Read the model definition and answer for the solid it produces. Units are mm, in the model's axes. A direction names the side the tool comes from. Round coordinates to 2 decimals unless told otherwise and drop trailing zeros. Order: outer loops, then holes, each group sorted by start corner. A loop starts at its lowest first (then second) coordinate and runs counter-clockwise, first axis right, second up. Notation, with made-up numbers: (4, 19.25) -> (63, 19.25) arc R5 cw to (63, 23.25) -> close; hole circle Ø8 at (-31.5, 15.25). An arc over 180 degrees is marked (long way). One line per item, written item: value. Start each with the question number.
1. Section D-D (z = 17.25) is taken. Give the vertices of the cut face in (x, y).
2. Section A-A (z = 5) is taken. Give the vertices of the cut face in (x, y) (3 decimals), then the cut area to 3 significant figures.
3. Section B-B (y = -2) is taken. Give the vertices of the cut face in (x, z), then the cut area to 3 significant figures.
4. For faces 5 (the face through (62, -6, 3)), 6 (the face through (35, -5, 0)), determine the directions among +Z, -Z, +X, -X, +Y, -Y from which every point of the face is accessible in a straight line to the end or side of a thin tool.
5. Consider line 1 (Z direction, x = 20, y = -9.1) (3 decimals); line 2 (Z direction, x = 60, y = -2.8); line 3 (X direction, y = -9, z = 3.25). Determine where each line is inside the solid, lowest interval first.
6. Section C-C (x = 60) is taken. Give the vertices of the cut face in (y, z) (3 decimals).
7. Flat-ended cylindrical pins translate along their axes: pin 1 Ø7 at (x, z) = (20, 5) entering from -Y; pin 2 Ø1.5 at (y, z) = (-3.5, 11.5) entering from +X; pin 3 Ø2.5 at (x, z) = (60, 5) entering from +Y. Find the tip coordinate at first contact, or state that the pin passes through.
8. The mould has two halves that part along X. Classify faces 1 (the face through (17.968, -2.958, 4.157)), 2 (the face through (0, -5, 10)), 3 (the face through (39, 0, 10)), 4 (the face through (15.88, -8.03, 5.18)): released by +X, released by -X, zero draft, split by the parting line, or undercut.
from build123d import *

# Parameters (mm, degrees)
F1_DEPTH       = 10
F3_D           = 4.4
F3_CBORE_D     = 8.25
F3_CBORE_DEPTH = 4


# Not quite as in the source:
# - a feature names something its author has since deleted; it is built from what else it names


with BuildPart() as f1:
    # F0 (on Front) → F1 (new body)
    with BuildSketch(Plane.XZ):
        Polygon((0, 10), (0, 0), (70, 0), (80, 10), align=None)
        Polygon((0, 20), (0, 10), (80, 10), (70, 20), align=None)
    extrude(amount=F1_DEPTH)

    # F3 (through all)
    with Locations(Plane.XZ.offset(10)):
        with Locations((20, 5), (60, 5)):
            CounterBoreHole(F3_D / 2, F3_CBORE_D / 2, F3_CBORE_DEPTH)


solid = f1.part
Answer:
1. outline: (0, -10) -> (72.75, -10) -> (72.75, 0) -> (0, 0) -> close
2. outline: (0, -10) -> (15.875, -10) -> (15.875, -6) -> (17.8, -6) -> (17.8, 0) -> (0, 0) -> close; (22.2, -6) -> (24.125, -6) -> (24.125, -10) -> (55.875, -10) -> (55.875, -6) -> (57.8, -6) -> (57.8, 0) -> (22.2, 0) -> close; (62.2, -6) -> (64.125, -6) -> (64.125, -10) -> (75, -10) -> (75, 0) -> (62.2, 0) -> close
2. area: 631 mm^2
3. outline: (0, 0) -> (70, 0) -> (80, 10) -> (70, 20) -> (0, 20) -> close; hole circle Ø4.4 at (20, 5); hole circle Ø4.4 at (60, 5)
3. area: 1,470 mm^2
4. face 5: -Y
4. face 6: -Z, +X, -X, +Y, -Y
5. line 1: 0 to 0.875, 9.125 to 20
5. line 2: 0 to 2.8, 7.2 to 20
5. line 3: 0 to 16.26, 23.74 to 56.26, 63.74 to 73.25
6. outline: (-10, 0) -> (0, 0) -> (0, 2.8) -> (-6, 2.8) -> (-6, 0.875) -> (-10, 0.875) -> close; (-10, 9.125) -> (-6, 9.125) -> (-6, 7.2) -> (0, 7.2) -> (0, 20) -> (-10, 20) -> close
7. pin 1: y = -6
7. pin 2: x = 79.25
7. pin 3: through
8. face 1: undercut
8. face 2: released by -X
8. face 3: zero draft
8. face 4: undercut
